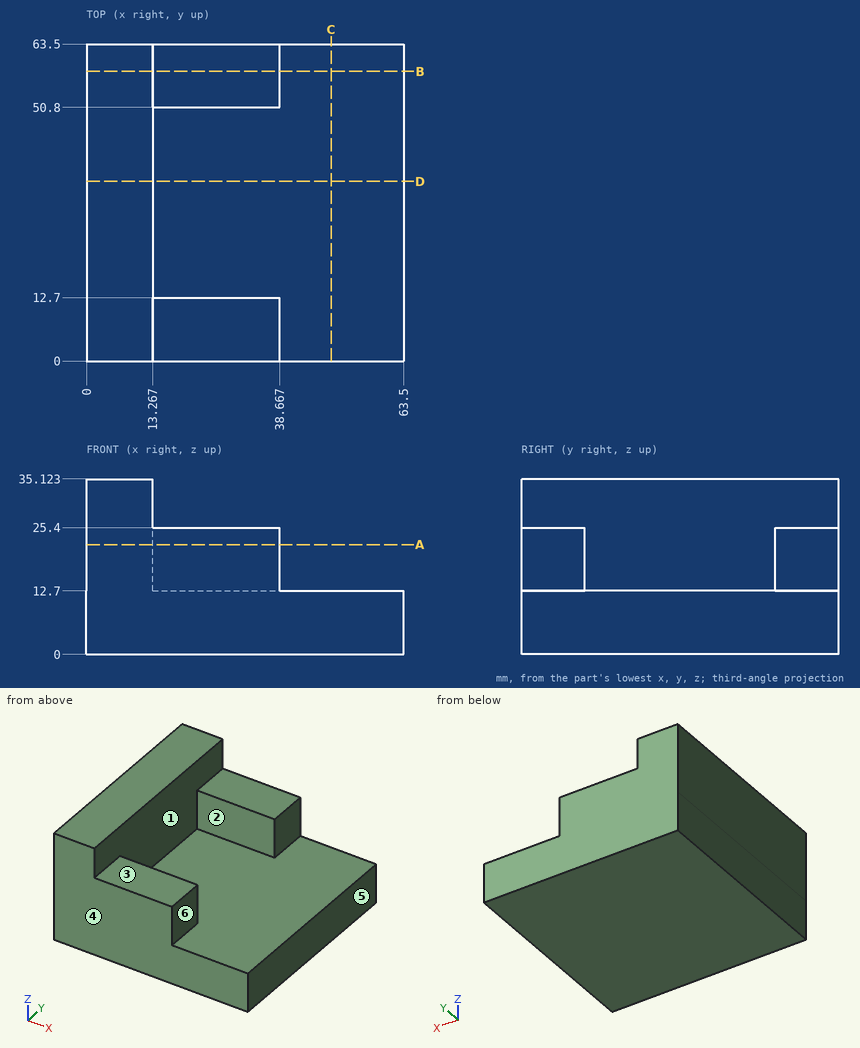
Source: three-view drawing plus pictorial views. Frame: mm from the lowest corner of the part. A direction names the side the tool comes from. Coordinates: 2 decimals unless noted, no trailing zeros. Loops run counter-clockwise (first coordinate to the right, second up) from the corner with the lowest first, then second, coordinate; pieces in that order, holes last. Notation, with made-up numbers: (19, 81) -> (49, 81) arc R18 ccw to (49, 90) -> close; hole circle Ø10 at (-35.5, -25.5). An arc over 180 degrees is marked (long way). Write each question's results on one line, items separated by ' | '. Start each with the question number.
Q1. Section B-B, the plane y = 58. Return the cut outline in (x, z).
Q2. Pull-direction query (Y, two-part tool) for the marked faces 1, 2, 3 and 4; classes: released by +Y, released by -Y, zero draft, split by the parting line, or undercut.
Q3. Pin query (flat end, axial travel): pin 1 (10 mm diameter, centred on y = 58.5, z = 20.5, fed in from +X); pin 2 (1.5 mm diameter, centred on x = 48.5, y = 13, fed in from +Z); pin 3 (4 mm diameter, centred on x = 29, y = 55.5, fed in from +Z). Return the tip coordinate at first contact, or that it passes through.
Q4. Section D-D, the plane y = 36. Return the cut outline in (x, z), plus the area to 3 significant figures.
Q5. Ray query, line 1 (Y direction, x = 19, z = 25); line 2 (Z direction, x = 20, y = 10.5); line 3 (X direction, y = 59, z = 30). Return the intervals inside material, ascending. Write a range as from..to.
Q6. Reachability of the marked faces 5 and 6 from +Z, -Z, +X, -X, +Y, -Y: full face, straight path, thin tool, end or side. Return the list, or none.
Q7. Section C-C, the plane x = 49. Return the cut outline in (y, z).
Q8. Section A-A, the plane z = 22. Return the cut outline in (x, y), plus the area to 3 significant figures.
Found:
1) outline: (0, 0) -> (63.5, 0) -> (63.5, 12.7) -> (38.67, 12.7) -> (38.67, 25.4) -> (13.27, 25.4) -> (13.27, 35.12) -> (0, 35.12) -> close
2) face 1: undercut | face 2: undercut | face 3: zero draft | face 4: released by -Y
3) pin 1: x = 38.67 | pin 2: z = 12.7 | pin 3: z = 25.4
4) outline: (0, 0) -> (63.5, 0) -> (63.5, 12.7) -> (13.27, 12.7) -> (13.27, 35.12) -> (0, 35.12) -> close | area: 1,100 mm2
5) line 1: 0..12.7, 50.8..63.5 | line 2: 0..25.4 | line 3: 0..13.27
6) face 5: +Z, -Z, +X, +Y, -Y | face 6: +Z, +X, +Y, -Y
7) outline: (0, 0) -> (63.5, 0) -> (63.5, 12.7) -> (0, 12.7) -> close
8) outline: (0, 0) -> (38.67, 0) -> (38.67, 12.7) -> (13.27, 12.7) -> (13.27, 50.8) -> (38.67, 50.8) -> (38.67, 63.5) -> (0, 63.5) -> close | area: 1,490 mm2
